Read the model definition and answer for the solid it produces. Units are mm, in the model's axes. A direction names the side the tool comes from. Give positions to 0.01 mm unless a question says otherwise; leave off trailing zeros. Write each loop counter-clockwise with the first axis right and the second up, starting at its lowest first coordinate (ties: lowest second). Pieces come first, ordered by that corner, then holes.
```python
from build123d import *

# Parameters (mm, degrees)
SKETCH1_W               = 15
SKETCH1_H               = 13
BASE_DEPTH              = 0.3
SKETCH2_R               = 4
PT_CUT_DEPTH            = 10.92924972
WIRE_CONNECTION_DEPTH   = 1
SKETCH7_W               = 1.8
SKETCH7_H               = 2.4
LOCKING_CLAMP_CUT_DEPTH = 11.816191566
LOCKING_CLAMP_DEPTH     = 0.8
SKETCH9_W               = 9
SKETCH9_H               = 2
BOTTOM_SLOT_CUT_DEPTH   = 11.816191566
TS_F_R                  = 1
BS_F_R                  = 4
WC_F_R                  = 0.5
BSC_F_R                 = 0.4


with BuildPart() as part:
    # Sketch1 → BASE (new body)
    with BuildSketch(Plane(origin=(0, 0, 0), x_dir=(1, 0, 0), z_dir=(0, 1, 0))):
        Rectangle(SKETCH1_W, SKETCH1_H)
    extrude(amount=BASE_DEPTH)

    # Sketch2 → PT CUT (cut, through all)
    with BuildSketch(Plane(origin=(0, 0.3, 0), x_dir=(1, 0, 0), z_dir=(0, 1, 0))):
        with Locations(Location((0, -1.9, 0), (0, 0, 270))):
            Circle(SKETCH2_R)
    extrude(amount=-PT_CUT_DEPTH, mode=Mode.SUBTRACT)

    # Sketch4 → POSITIVE TERMINAL (revolve)
    with BuildSketch(Plane.XY.offset(1.9), mode=Mode.PRIVATE) as positive_terminal_sk:
        with BuildLine():
            Line((0, 2.6), (1.056776663, 2.6))
            ThreePointArc((1.056776663, 2.6), (1.191616938, 2.576587441), (1.310672433, 2.509090502))
            Line((1.310672433, 2.509090502), (4, 0.3))
            Line((4, 0.3), (4, 0))
            Line((4, 0), (3.7, 0))
            ThreePointArc((3.7, 0), (3.629289322, 0.029289322), (3.6, 0.1))
            Line((3.6, 0.1), (3.6, 0.252730922))
            ThreePointArc((3.6, 0.252730922), (3.590408501, 0.295466187), (3.563473942, 0.330003547))
            Line((3.563473942, 0.330003547), (1.220553608, 2.254545251))
            ThreePointArc((1.220553608, 2.254545251), (1.16102586, 2.28829372), (1.093605723, 2.3))
            Line((1.093605723, 2.3), (0, 2.3))
            Line((0, 2.3), (0, 2.6))
        make_face()
    revolve(positive_terminal_sk.sketch.rotate(Axis((0, 0, 1.9), (0, 1, 0)), 90), axis=Axis((0, 0, 1.9), (0, 1, 0)))

    # Sketch5 → WIRE CONNECTION (add, symmetric)
    with BuildSketch(Plane(origin=(0, 0, 0), x_dir=(0, 0, -1), z_dir=(1, 0, 0))):
        Polygon((-6.5, 0), (-2.5, -4), (-2.2, -4), (-6.2, 0), align=None)
    extrude(amount=WIRE_CONNECTION_DEPTH, both=True)

    # Sketch7 → LOCKING CLAMP CUT (cut, through all)
    with BuildSketch(Plane(origin=(0, 0.3, 0), x_dir=(1, 0, 0), z_dir=(0, 1, 0))):
        with Locations((6.2, -0.3)):
            Rectangle(SKETCH7_W, SKETCH7_H)
    locking_clamp_cut = extrude(amount=-LOCKING_CLAMP_CUT_DEPTH, mode=Mode.SUBTRACT)

    # Sketch8 → LOCKING CLAMP (add, symmetric)
    with BuildSketch(Plane(origin=(6.2, 0, 0), x_dir=(0, 0, -1), z_dir=(1, 0, 0))):
        Polygon((0.9, -1), (-1.5, 0.3), (-1.5, 0), (0.9, -1.3), align=None)
    locking_clamp = extrude(amount=LOCKING_CLAMP_DEPTH, both=True)

    # LC M: LOCKING CLAMP CUT, LOCKING CLAMP across plane
    add(locking_clamp_cut.mirror(Plane(origin=(0, 0, 0), x_dir=(0, 0, 1), z_dir=(1, 0, 0))), mode=Mode.SUBTRACT)
    add(locking_clamp.mirror(Plane(origin=(0, 0, 0), x_dir=(0, 0, 1), z_dir=(1, 0, 0))))

    # Sketch9 → BOTTOM SLOT CUT (cut, through all)
    with BuildSketch(Plane(origin=(0, 0.3, 0), x_dir=(1, 0, 0), z_dir=(0, 1, 0))):
        with Locations((0, 5.5)):
            Rectangle(SKETCH9_W, SKETCH9_H)
    extrude(amount=-BOTTOM_SLOT_CUT_DEPTH, mode=Mode.SUBTRACT)

    # TS F
    ts_f_edges = [part.edges().sort_by_distance(p)[0] for p in [
        (-7.5, 0.15, -6.5),
        (7.5, 0.15, -6.5),
    ]]
    fillet(ts_f_edges, radius=TS_F_R)

    # BS F
    bs_f_edges = [part.edges().sort_by_distance(p)[0] for p in [
        (7.5, 0.15, 6.5),
        (-7.5, 0.15, 6.5),
    ]]
    fillet(bs_f_edges, radius=BS_F_R)

    # WC F
    # the kernel refuses this fillet: 0.5 mm, written as the material it takes off along each edge
    with BuildSketch(Plane(origin=(-1, -4, 3.75), x_dir=(0, 1, 0), z_dir=(0, 0, -1))) as wc_f_piece_1:
        with BuildLine():
            CenterArc((WC_F_R, WC_F_R), WC_F_R, 180, 90)
            Line((0, WC_F_R), (0, 0))
            Line((0, 0), (WC_F_R, 0))
        make_face()
    extrude(amount=2.8, mode=Mode.SUBTRACT)
    with BuildSketch(Plane(origin=(1, -4, 3.75), x_dir=(0, 1, 0), z_dir=(0, 0, -1))) as wc_f_piece_2:
        with BuildLine():
            CenterArc((WC_F_R, -WC_F_R), WC_F_R, 90, 90)
            Line((0, -WC_F_R), (0, 0))
            Line((0, 0), (WC_F_R, 0))
        make_face()
    extrude(amount=2.8, mode=Mode.SUBTRACT)

    # BSC F
    bsc_f_edges = [part.edges().sort_by_distance(p)[0] for p in [
        (-4.5, 0.15, -6.5),
        (4.5, 0.15, -6.5),
        (4.5, 0.15, -4.5),
        (-4.5, 0.15, -4.5),
    ]]
    fillet(bsc_f_edges, radius=BSC_F_R)


solid = part.part
```
Item 1: Determine the mould class of faces 1 (the flat face through (0, 2.3, 2)), 2 (the flat face through (-6.21, -0.64, 0.32)), 3 (the flat face through (6.21, -0.36, 0.28)) for opening direction Y: pulls with the +Y half, pulls with the -Y half, needs draft (parallel to the pull), parting line crosses it, or undercut.
Result set:
face 1: undercut
face 2: pulls with the -Y half
face 3: pulls with the +Y half
Item 2: Which of the six approach directions +Z, -Z, +X, -X, +Y, -Y give full straight-line access (tool end or side, diameter ignored) to faces 4 (the flat face through (0, -2, 4.2)), 5 (the flat face through (6.21, -0.64, 0.32)), 6 (the flat face through (-6.21, -0.36, 0.28))?
Result set:
face 4: -Z, +X, -X
face 5: +Z, +X, -X, -Y
face 6: +Y
Item 3: Section D-D (y = 0.75) is taken. Write down the section's boundary in (x, z).
Result set:
outline: circle Ø6.9 at (0, 1.9); hole circle Ø6.1 at (0, 1.9)
Item 4: Each of these flat-tipped pins is pushed along its axis until it touches: pin 1 Ø0.8 at (y, z) = (-0.5, 0) entering from +X; pin 2 Ø2 at (y, z) = (-3.5, 2.5) entering from +X; pin 3 Ø1.5 at (y, z) = (1.5, -2) entering from +X; pin 4 Ø0.7 at (x, z) = (-0.5, 1.5) entering from -Y. Where does it stop, or does it pass through?
Result set:
pin 1: stops at x = 7
pin 2: stops at x = 1
pin 3: passes through
pin 4: stops at y = 2.3
Item 5: Section B-B (z = 1.9) is taken. Write down the section's boundary in (x, y).
Result set:
outline: (-7.5, 0) - (-3.7, 0) arc R0.1 ccw to (-3.6, 0.1) - (-3.6, 0.25) arc R0.1 cw to (-3.56, 0.33) - (-1.22, 2.25) arc R0.2 cw to (-1.09, 2.3) - (1.09, 2.3) arc R0.2 cw to (1.22, 2.25) - (3.56, 0.33) arc R0.1 cw to (3.6, 0.25) - (3.6, 0.1) arc R0.1 ccw to (3.7, 0) - (7.5, 0) - (7.5, 0.3) - (4, 0.3) - (1.31, 2.51) arc R0.4 ccw to (1.06, 2.6) - (-1.06, 2.6) arc R0.4 ccw to (-1.31, 2.51) - (-4, 0.3) - (-7.5, 0.3) - close
Item 6: Section A-A (x = 6.25) is taken. Write down the section's boundary in (y, z), and give its area (3 significant figures).
Result set:
outline: (-1.3, -0.9) - (-1, -0.9) - (0.3, 1.5) - (0.3, 5.4) - (0, 5.4) - (0, 1.5) - close; (0, -6.5) - (0.3, -6.5) - (0.3, -0.9) - (0, -0.9) - close
area: 3.57 mm2
Item 7: Find the intervals of material crossed by line 1 along X through (y, z) = (0.2, 1.9); line 2 along Y through (x, z) = (-5, 4.75); line 3 along Y through (x, z) = (0.5, 3.25), in increasing order.
Result set:
line 1: x = -7.5 to -3.6, 3.6 to 7.5
line 2: y = 0 to 0.3
line 3: y = -3.25 to -2.95, 2.07 to 2.4
Item 8: Section C-C (x = 0) is taken. Write down the section's boundary in (y, z).
Result set:
outline: (-4, 2.2) - (0, 6.2) - (0, 5.6) arc R0.1 ccw to (0.1, 5.5) - (0.25, 5.5) arc R0.1 cw to (0.33, 5.46) - (2.25, 3.12) arc R0.2 cw to (2.3, 2.99) - (2.3, 0.81) arc R0.2 cw to (2.25, 0.68) - (0.33, -1.66) arc R0.1 cw to (0.25, -1.7) - (0.1, -1.7) arc R0.1 ccw to (0, -1.8) - (0, -4.5) - (0.3, -4.5) - (0.3, -2.1) - (2.51, 0.59) arc R0.4 ccw to (2.6, 0.84) - (2.6, 2.96) arc R0.4 ccw to (2.51, 3.21) - (0.3, 5.9) - (0.3, 6.5) - (0, 6.5) - (-4, 2.5) - close
